Verification items for the finished model (mm, model axes). Face numbers are marked on the shaded views. A direction names the side the tool comes from. Coordinates: 2 decimals unless noted, no trailing zeros. Order: outer loops, then holes, each group sorted by start corner. A loop starts at its lowest first (then second) coordinate and runs counter-clockwise, first axis right, second up. Notation, with made-up numbers: (-3.5, 73.25) -> (22.5, 73.25) arc R35 ccw to (22.5, 107.25) -> close; hole circle Ø6 at (3, 27). An arc over 180 degrees is marked (long way). Answer as CSV lines item,"result".
```python
from build123d import *

# Parameters (mm, degrees)
SKETCH_1_W          = 43
SKETCH_1_H          = 43.5
SKETCH_1_R          = 1.5
EXTRUDE_1_DEPTH     = 2
SKETCH_2_W          = 15.5
SKETCH_2_H          = 26
EXTRUDE_2_DEPTH     = 25
SKETCH_3_W          = 10.4
SKETCH_3_H          = 24
SKETCH_3_W_2        = 3.4
SKETCH_3_H_2        = 0.926804748
SKETCH_3_H_3        = 0.774498031
SKETCH_3_H_4        = 2.236086948
SKETCH_3_H_5        = 3.79712878
SKETCH_3_H_6        = 1.178452045
SKETCH_3_H_7        = 1.322605193
SKETCH_3_H_8        = 1.93303836
SKETCH_3_H_9        = 2.068690175
CUT_EXTRUDE_1_DEPTH = 25


with BuildPart() as part:
    # 草图1 → 凸台-拉伸1 (new body)
    with BuildSketch(Plane.XY):
        Rectangle(SKETCH_1_W, SKETCH_1_H)
        with Locations((-18.5, 18.431705674)):
            Circle(SKETCH_1_R, mode=Mode.SUBTRACT)
        with Locations(Location((18.5, -18.431705674, 0), (0, 0, 180))):
            Circle(SKETCH_1_R, mode=Mode.SUBTRACT)
        with Locations(Location((-18.5, -18.431705674, 0), (0, 0, 180))):
            Circle(SKETCH_1_R, mode=Mode.SUBTRACT)
        with Locations((18.5, 18.431705674)):
            Circle(SKETCH_1_R, mode=Mode.SUBTRACT)
    extrude(amount=EXTRUDE_1_DEPTH)

    # 草图2 → 凸台-拉伸2 (add)
    with BuildSketch(Plane.XY.offset(2)):
        with Locations((12.25, 0)):
            Rectangle(SKETCH_2_W, SKETCH_2_H)
    extrude(amount=EXTRUDE_2_DEPTH)

    # 草图3 → 切除-拉伸1 (cut)
    with BuildSketch(Plane.XY.offset(27)):
        with Locations((9.7, 0)):
            Rectangle(SKETCH_3_W, SKETCH_3_H)
        with Locations((18.3, 11.536597626)):
            Rectangle(SKETCH_3_W_2, SKETCH_3_H_2)
        with Locations((18.3, -11.612750984)):
            Rectangle(SKETCH_3_W_2, SKETCH_3_H_3)
        with Locations((18.3, 7.69685645)):
            Rectangle(SKETCH_3_W_2, SKETCH_3_H_4)
        with Locations((18.3, 4.131774429)):
            Rectangle(SKETCH_3_W_2, SKETCH_3_H_5)
        with Locations((18.3, 0.589226023)):
            Rectangle(SKETCH_3_W_2, SKETCH_3_H_6)
        with Locations((18.3, -9.727346991)):
            Rectangle(SKETCH_3_W_2, SKETCH_3_H_7)
        with Locations((18.3, -7.285614326)):
            Rectangle(SKETCH_3_W_2, SKETCH_3_H_8)
        with Locations((18.3, -4.267361447)):
            Rectangle(SKETCH_3_W_2, SKETCH_3_H_9)
    extrude(amount=-CUT_EXTRUDE_1_DEPTH, mode=Mode.SUBTRACT)


solid = part.part
```
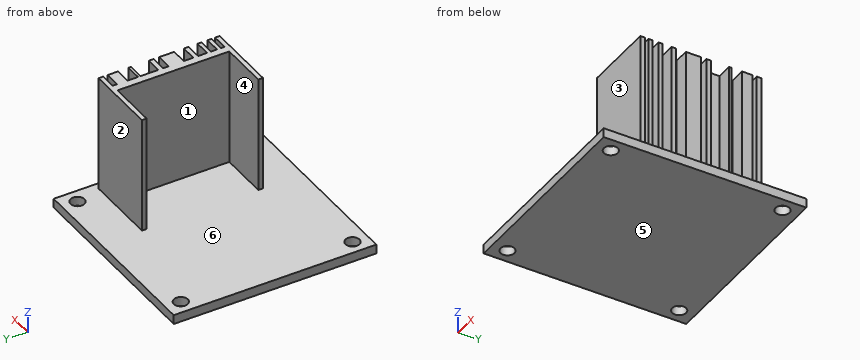
Item 1: Thickness scan on line 1 (Y direction, x = 18.5, z = 0.95); line 2 (Y direction, x = 10, z = 9.75); line 3 (Z direction, x = 9, y = 18). Record the ranges inside material, lowest first.
Answer list:
line 1,"-21.75 to -19.93, -16.93 to 16.93, 19.93 to 21.75"
line 2,"-13 to -12, 12 to 13"
line 3,"0 to 2"
Item 2: Release check for a two-part mould opening along Y. For the marked faces 3, 4, 5 and 6 record: +Y half, -Y half, draft (parallel to the pull), parting line (faces both ways), or undercut.
Answer list:
face 3,"-Y half"
face 4,"undercut"
face 5,"draft"
face 6,"undercut"
Item 3: Tool access check on the marked faces 1 and 2. Record the directions out of +Z, -Z, +X, -X, +Y, -Y that give a thin tool (end or side, any length) a straight path to the whole face; none if there is none.
Answer list:
face 1,"+Z, -X"
face 2,"+Z, +X, -X, +Y"
Item 4: Depth check by flat-ended pin: pin 1 Ø1.8 at (x, y) = (-18.5, -18.43) entering from +Z; pin 2 Ø1.7 at (x, z) = (18.5, 11) entering from -Y; pin 3 Ø3 at (y, z) = (13, 4) entering from -X; pin 4 Ø0.5 at (y, z) = (-12.5, 11) entering from +X. Enter the tip coordinate at first touch or a pass-through.
Answer list:
pin 1,"through"
pin 2,"y = -13"
pin 3,"x = 4.5"
pin 4,"x = 20"
Item 5: Section check C-C, the plane x = 18.5. Count the separate pieces of the cut face and the enclosed holes in it, plus the area to 3 significant figures.
Answer list:
separate pieces,"3"
enclosed holes,"0"
area,"369 mm2"
Item 6: Section check A-A, the plane x = -18.5. Record the boundary of the cut face in (y, z), plus the area to 3 significant figures.
Answer list:
outline,"(-21.75, 0) -> (-19.93, 0) -> (-19.93, 2) -> (-21.75, 2) -> close; (-16.93, 0) -> (16.93, 0) -> (16.93, 2) -> (-16.93, 2) -> close; (19.93, 0) -> (21.75, 0) -> (21.75, 2) -> (19.93, 2) -> close"
area,"75.0 mm2"
Item 7: Section check B-B, the plane x = -13. Record the boundary of the cut face in (y, z), plus the area to 3 significant figures.
Answer list:
outline,"(-21.75, 0) -> (21.75, 0) -> (21.75, 2) -> (-21.75, 2) -> close"
area,"87.0 mm2"
